Could you check a few things on this model? Use its own coordinates, in mm. Round coordinates to 2 decimals unless told otherwise and drop trailing zeros. Loops run counter-clockwise (first coordinate to the right, second up) from the corner with the lowest first, then second, coordinate; pieces in that order, holes last. Notation, with made-up numbers: (70.25, 88.25) -> (106.25, 88.25) arc R27 ccw to (106.25, 120.25) -> close; hole circle Ø9 at (6, 75). An arc over 180 degrees is marked (long way). Write each question's results on one line, items separated by ' | '. Start each with the question number.
1) Imagine slicing it at C-C, the plane y = 0. Give the number of separate pieces and of enclosed holes in the cut face, plus the area to 3 significant figures.
2) Imagine slicing it at B-B, the plane z = 1.5. List the corners of the cut face in (x, y) for me, plus the area to 3 significant figures.
3) Imagine slicing it at A-A, the plane x = 1.27. List the corners of the cut face in (y, z) for me.
4) If I drill on probe 1 along X at (y, z) = (-0.15, 4.25); probe 2 along Y at (x, z) = (-1.27, 8.8); probe 3 along Y at (x, z) = (-3.75, 2.5), over which ranges is the centre line in solid material (lowest first)?
5) Imagine slicing it at D-D, the plane z = 10.75. List the corners of the cut face in (x, y) for me.
from build123d import *

# Parameters (mm, degrees)
SKETCH_5_W      = 10
SKETCH_5_H      = 4
SKETCH_5_W_2    = 0.7
SKETCH_5_H_2    = 0.7
EXTRUDE_2_DEPTH = 8
SKETCH_6_W      = 10
SKETCH_6_H      = 4
SKETCH_6_R      = 0.5
EXTRUDE_3_DEPTH = 3
CHAMFER_3_SIZE  = 1


with BuildPart() as part:
    # Эскиз5 → Бобышка-Вытянуть2 (new body)
    with BuildSketch(Plane.XY):
        Rectangle(SKETCH_5_W, SKETCH_5_H)
        with Locations((-3.81, 0)):
            Rectangle(SKETCH_5_W_2, SKETCH_5_H_2, mode=Mode.SUBTRACT)
        with Locations((3.81, 0)):
            Rectangle(SKETCH_5_W_2, SKETCH_5_H_2, mode=Mode.SUBTRACT)
        with Locations((-1.27, 0)):
            Rectangle(SKETCH_5_W_2, SKETCH_5_H_2, mode=Mode.SUBTRACT)
        with Locations((1.27, 0)):
            Rectangle(SKETCH_5_W_2, SKETCH_5_H_2, mode=Mode.SUBTRACT)
    extrude(amount=EXTRUDE_2_DEPTH)

    # Эскиз6 → Бобышка-Вытянуть3 (add)
    with BuildSketch(Plane.XY.offset(8)):
        Rectangle(SKETCH_6_W, SKETCH_6_H)
        with Locations((-3.81, 0)):
            Circle(SKETCH_6_R, mode=Mode.SUBTRACT)
        with Locations((-1.27, 0)):
            Circle(SKETCH_6_R, mode=Mode.SUBTRACT)
        with Locations((1.27, 0)):
            Circle(SKETCH_6_R, mode=Mode.SUBTRACT)
        with Locations((3.81, 0)):
            Circle(SKETCH_6_R, mode=Mode.SUBTRACT)
    extrude(amount=EXTRUDE_3_DEPTH)

    # Фаска3
    chamfer_3_edges = [part.edges().sort_by_distance(p)[0] for p in [
        (5, -2, 5.5),
        (-5, -2, 5.5),
        (-5, 2, 5.5),
        (5, 2, 5.5),
    ]]
    chamfer(chamfer_3_edges, length=CHAMFER_3_SIZE)


solid = part.part
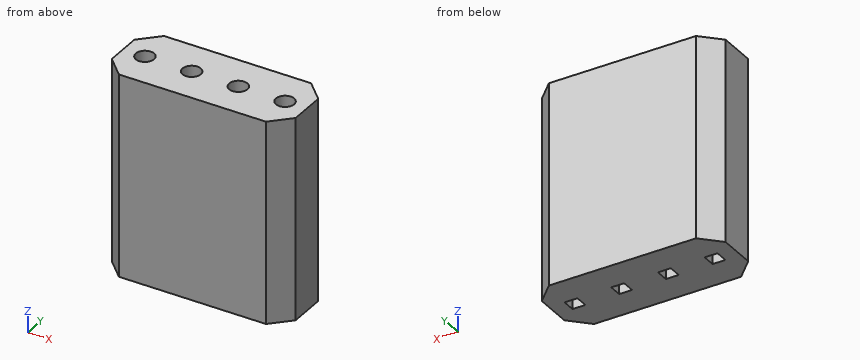
Checked values:
1) separate pieces: 5 | enclosed holes: 0 | area: 75.6 mm^2
2) outline: (-5, -1) -> (-4, -2) -> (4, -2) -> (5, -1) -> (5, 1) -> (4, 2) -> (-4, 2) -> (-5, 1) -> close; hole (-4.16, -0.35) -> (-3.46, -0.35) -> (-3.46, 0.35) -> (-4.16, 0.35) -> close; hole (-1.62, -0.35) -> (-0.92, -0.35) -> (-0.92, 0.35) -> (-1.62, 0.35) -> close; hole (0.92, -0.35) -> (1.62, -0.35) -> (1.62, 0.35) -> (0.92, 0.35) -> close; hole (3.46, -0.35) -> (4.16, -0.35) -> (4.16, 0.35) -> (3.46, 0.35) -> close | area: 36.0 mm^2
3) outline: (-2, 0) -> (-0.35, 0) -> (-0.35, 8) -> (-0.5, 8) -> (-0.5, 11) -> (-2, 11) -> close; (0.35, 0) -> (2, 0) -> (2, 11) -> (0.5, 11) -> (0.5, 8) -> (0.35, 8) -> close
4) probe 1: -5 to -4.16, -3.46 to -1.62, -0.92 to 0.92, 1.62 to 3.46, 4.16 to 5 | probe 2: -2 to -0.5, 0.5 to 2 | probe 3: -2 to -0.35, 0.35 to 2
5) outline: (-5, -1) -> (-4, -2) -> (4, -2) -> (5, -1) -> (5, 1) -> (4, 2) -> (-4, 2) -> (-5, 1) -> close; hole circle Ø1 at (-3.81, 0); hole circle Ø1 at (-1.27, 0); hole circle Ø1 at (1.27, 0); hole circle Ø1 at (3.81, 0)
